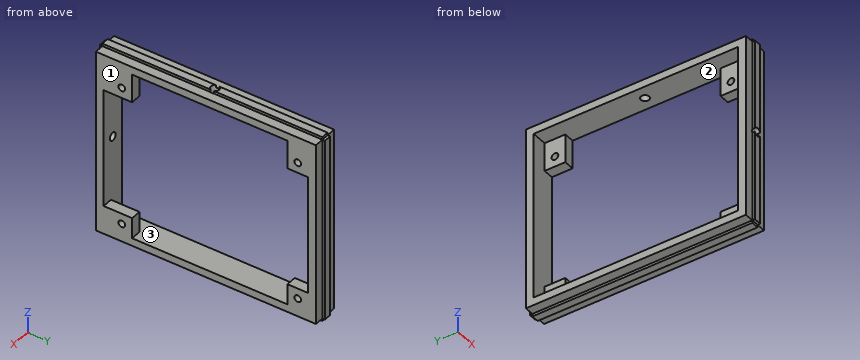
```python
from build123d import *

# Parameters (mm, degrees)
MAIN_DEPTH           = 71
SKETCH2_W            = 2.9
SKETCH2_H            = 85
MAKERBEAMRAIL1_DEPTH = 1
SKETCH3_W            = 2.9
SKETCH3_H            = 85
MAKERBEAMRAIL2_DEPTH = 1
SKETCH4_W            = 65
SKETCH4_H            = 79
BOARDCUT_DEPTH       = 6
SKETCH5_R            = 1.3
BOARDHOLES_DEPTH     = 5
SKETCH6_R            = 1.6
FIXHOLE1_DEPTH       = 4
MAINHOLE_DEPTH       = 5
FIXHOLE2_REACH       = 89
SKETCH8_R            = 1.6


with BuildPart() as part:
    # Sketch1 → Main (new body)
    with BuildSketch(Plane.XY):
        Polygon((0, 85), (3.55, 85), (3.55, 86), (6.45, 86), (6.45, 85), (10, 85), (10, 0), (6.45, 0), (6.45, -1), (3.55, -1), (3.55, 0), (0, 0), align=None)
    extrude(amount=MAIN_DEPTH)

    # Sketch2 → MakerBeamRail1 (add)
    with BuildSketch(Plane.XY.offset(71)):
        with Locations((5, 42.5)):
            Rectangle(SKETCH2_W, SKETCH2_H)
    extrude(amount=MAKERBEAMRAIL1_DEPTH)

    # Sketch3 → MakerBeamRail2 (add)
    with BuildSketch(Plane(origin=(0, 0, 0), x_dir=(-1, 0, 0), z_dir=(0, 0, -1))):
        with Locations((-5, 42.5)):
            Rectangle(SKETCH3_W, SKETCH3_H)
    extrude(amount=MAKERBEAMRAIL2_DEPTH)

    # Sketch4 → BoardCut (cut)
    with BuildSketch(Plane.ZY):
        with Locations((35.5, 42.5)):
            Rectangle(SKETCH4_W, SKETCH4_H)
    extrude(amount=-BOARDCUT_DEPTH, mode=Mode.SUBTRACT)

    # Sketch5 → BoardHoles (cut, through all)
    with BuildSketch(Plane.ZY.offset(-6)):
        with Locations((7, 78)):
            Circle(SKETCH5_R)
        with Locations((61, 78)):
            Circle(SKETCH5_R)
        with Locations((61, 10)):
            Circle(SKETCH5_R)
        with Locations((7, 10)):
            Circle(SKETCH5_R)
    extrude(amount=-BOARDHOLES_DEPTH, mode=Mode.SUBTRACT)

    # Sketch6 → FixHole1 (cut)
    with BuildSketch(Plane.XY.offset(72)):
        with Locations((5, 42.5)):
            Circle(SKETCH6_R)
    extrude(amount=-FIXHOLE1_DEPTH, mode=Mode.SUBTRACT)

    # Sketch7 → MainHole (cut, through all)
    with BuildSketch(Plane.ZY.offset(-6)):
        Polygon((3, 74), (11, 74), (11, 82), (57, 82), (57, 74), (68, 74), (68, 14), (57, 14), (57, 3), (11, 3), (11, 14), (3, 14), align=None)
    extrude(amount=-MAINHOLE_DEPTH, mode=Mode.SUBTRACT)

    # Sketch8 → FixHole2 (cut, up to next)
    with BuildSketch(Plane(origin=(0, -1, 0), x_dir=(-1, 0, 0), z_dir=(0, -1, 0)), mode=Mode.PRIVATE) as fixhole2_sk1:
        with Locations((-5, -35.5)):
            Circle(SKETCH8_R)
    fixhole2_tool1 = extrude(fixhole2_sk1.sketch, amount=-FIXHOLE2_REACH, mode=Mode.PRIVATE) & part.part
    add(fixhole2_tool1.solids().sort_by_distance((5, -1, 35.5))[0], mode=Mode.SUBTRACT)


solid = part.part
```
Input: part model. Units: mm. Frame: model coordinates. Face numbers are marked on the shaded views. Give positions to 0.01 mm unless a question says otherwise; leave off trailing zeros. Order: outer loops, then holes, each group sorted by start corner. A loop starts at its lowest first (then second) coordinate and runs counter-clockwise, first axis right, second up. Notation, with made-up numbers: M -2,-32.75 L 30,-32.75 A26 ccw 30,-4.75 Z; hole C -18.5,31 d2. An arc over 180 degrees is marked long. One line per question, with ' | ' between items.
1) Section A-A on z = 7. Output: boundary loops of the cut face in (x, y).
Filled in:
outline: M 0,0 L 3.55,0 L 3.55,-1 L 6.45,-1 L 6.45,0 L 10,0 L 10,8.7 L 6,8.7 L 6,3 L 0,3 Z; M 0,82 L 6,82 L 6,79.3 L 10,79.3 L 10,85 L 6.45,85 L 6.45,86 L 3.55,86 L 3.55,85 L 0,85 Z; M 6,11.3 L 10,11.3 L 10,14 L 6,14 Z; M 6,74 L 10,74 L 10,76.7 L 6,76.7 Z
2) Section D-D on z = 16.5. Output: boundary loops of the cut face in (x, y), and give its area (3 significant figures).
Filled in:
outline: M 0,0 L 3.55,0 L 3.55,-1 L 6.45,-1 L 6.45,0 L 10,0 L 10,3 L 0,3 Z; M 0,82 L 10,82 L 10,85 L 6.45,85 L 6.45,86 L 3.55,86 L 3.55,85 L 0,85 Z | area: 65.8 mm2
3) Ray query, L1, parallel to Y at x = 8.1, z = 61; L2, parallel to Z at x = 8.15, y = 78; L3, parallel to Z at x = 6, y = 24. Return the intervals inside material, ascending.
Filled in:
L1: y = 0 to 8.7, 11.3 to 14, 74 to 76.7, 79.3 to 85 | L2: z = 0 to 5.7, 8.3 to 11, 57 to 59.7, 62.3 to 71 | L3: z = -1 to 3, 68 to 72
4) Section B-B on y = 10. Output: boundary loops of the cut face in (x, z).
Filled in:
outline: M 0,0 L 3.55,0 L 3.55,-1 L 6.45,-1 L 6.45,0 L 10,0 L 10,5.7 L 6,5.7 L 6,3 L 0,3 Z; M 0,68 L 6,68 L 6,62.3 L 10,62.3 L 10,71 L 6.45,71 L 6.45,72 L 3.55,72 L 3.55,71 L 0,71 Z; M 6,8.3 L 10,8.3 L 10,11 L 6,11 Z; M 6,57 L 10,57 L 10,59.7 L 6,59.7 Z
5) Contact query for flat-ended pins moving along their axis: P1, Ø5.5, axis at y = 6, z = 63.5, coming from the -X side; P2, Ø0.5, axis at y = 85.5, z = 36.5, coming from the -X side; P3, Ø2.5, axis at x = 5, y = 42.5, coming from the +Z side; P4, Ø1.5, axis at x = 3, y = 20.5, coming from the +Z side. Output: stop coordinate, or through.
Filled in:
P1: stops at x = 6 | P2: stops at x = 3.55 | P3: stops at z = 3 | P4: stops at z = 72
6) Draft query along Z for the marked faces 1, 2 and 3. Return one class per face: pulls with the +Z half, pulls with the -Z half, needs draft (parallel to the pull), parting line crosses it, or undercut.
Filled in:
face 1: needs draft | face 2: undercut | face 3: undercut
7) Section C-C on x = 5. Output: boundary loops of the cut face in (y, z).
Filled in:
outline: M -1,0 L 0,0 L 0,-1 L 85,-1 L 85,0 L 86,0 L 86,71 L 85,71 L 85,72 L 44.1,72 L 44.1,68 L 82,68 L 82,3 L 3,3 L 3,33.9 L -1,33.9 Z; M -1,37.1 L 3,37.1 L 3,68 L 40.9,68 L 40.9,72 L 0,72 L 0,71 L -1,71 Z
